For this review, take the finished solid that the model builds, in its own axes (mm). Face numbers are marked on the shaded views. A direction names the side the tool comes from. Give positions to 0.01 mm unless a question says otherwise; leave off trailing zeros. Order: outer loops, then holes, each group sorted by start corner. A loop starts at its lowest first (then second) coordinate and runs counter-clockwise, first axis right, second up.
Item 1: Consider section A-A (y = 10.75). Give the boundary of the cut face in (x, z).
Item 2: Consider section B-B (z = -9). Give the boundary of the cut face in (x, y).
Item 3: For probe 1 along X at (y, z) = (8.25, -6.5); probe 2 along Y at (x, z) = (3.1, -9); probe 3 along Z at (x, y) = (7, 10.3), list the stretches that pass through material, from the lowest coordinate up.
Item 4: Consider section C-C (x = 7). Give the boundary of the cut face in (y, z).
Item 5: For P1, Ø3, axis at x = 8.5, z = -3, coming from the -Y side; P2, Ø1.5, axis at y = 3, z = -18, coming from the +X side; P3, Ø1.2, axis at x = 6.5, y = 7.5, coming from the -Z side; P4, Ø1.2, axis at y = 3.5, z = -4, coming from the -X side, all flat-tipped, find the tip position at first contact; note any pin that passes through.
Item 6: The part is to be moulded in two halves that separate along Z. For the marked faces 1, 2 and 3, say which applies: released by +Z, released by -Z, zero draft, split by the parting line, or undercut.
Item 7: Consider section D-D (y = 3.5). Give the boundary of the cut face in (x, z).
Item 8: Machinability: for the marked faces 4, 5 and 6, which of the approach directions +Z, -Z, +X, -X, +Y, -Y give a long, thin tool a straight path to every point of the face, cutting with its end or side? Answer none if there is none.
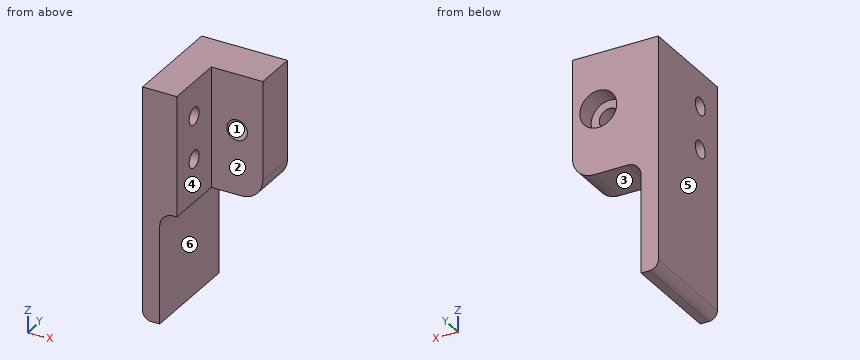
```python
from build123d import *

# Parameters (mm, degrees)
EXTRUDE_1_DEPTH              = 12
SKETCH_2_W                   = 6
SKETCH_2_H                   = 20
CUT_EXTRUDE_1_DEPTH          = 7
F_2_0MM_1_D                  = 2
HOLE_WIZARD_M2_1_D           = 2.4
HOLE_WIZARD_M2_1_CBORE_D     = 4.3
HOLE_WIZARD_M2_1_CBORE_DEPTH = 2.3


with BuildPart() as part:
    # 草图1 → 凸台-拉伸1 (new body)
    with BuildSketch(Plane(origin=(0, 0, 0), x_dir=(1, 0, 0), z_dir=(0, 1, 0))):
        with BuildLine():
            Line((3.6, 14), (7.5, 14))
            ThreePointArc((7.5, 14), (9.267766953, 13.267766953), (10, 11.5))
            Line((10, 11.5), (10, 0))
            Line((10, 0), (0, 0))
            Line((0, 0), (0, 26))
            ThreePointArc((0, 26), (0.292893219, 26.707106781), (1, 27))
            Line((1, 27), (2, 27))
            Line((2, 27), (2, 15.6))
            ThreePointArc((2, 15.6), (2.46862915, 14.46862915), (3.6, 14))
        make_face()
    extrude(amount=EXTRUDE_1_DEPTH)

    # 草图2 → 切除-拉伸1 (cut)
    with BuildSketch(Plane.XZ):
        with Locations((7, -10)):
            Rectangle(SKETCH_2_W, SKETCH_2_H)
    extrude(amount=-CUT_EXTRUDE_1_DEPTH, mode=Mode.SUBTRACT)

    # Ø2.0mm 暗销孔1 (through all)
    with Locations(Plane.ZY):
        with Locations((-4, 3.5), (-9, 3.5)):
            Hole(F_2_0MM_1_D / 2)

    # M2 六角圆柱头螺钉的柱形沉头孔1 (through all)
    with Locations(Plane(origin=(0, 12, 0), x_dir=(1, 0, 0), z_dir=(0, 1, 0))):
        with Locations((7, 6.5)):
            CounterBoreHole(HOLE_WIZARD_M2_1_D / 2, HOLE_WIZARD_M2_1_CBORE_D / 2, HOLE_WIZARD_M2_1_CBORE_DEPTH)


solid = part.part
```
Resolved:
1. outline: (0, -26) arc R1 ccw to (1, -27) - (2, -27) - (2, -15.6) arc R1.6 cw to (3.6, -14) - (7.5, -14) arc R2.5 ccw to (10, -11.5) - (10, 0) - (0, 0) - close; hole circle Ø4.3 at (7, -6.5)
2. outline: (0, 0) - (4, 0) - (4, 2.5) - (0, 2.5) - close; (0, 4.5) - (4, 4.5) - (4, 7) - (10, 7) - (10, 12) - (0, 12) - close
3. probe 1: x = 0 to 5.8, 8.2 to 10
3. probe 2: y = 0 to 2.5, 4.5 to 12
3. probe 3: z = -14 to -8.65, -4.35 to 0
4. outline: (7, -14) - (12, -14) - (12, -8.65) - (9.7, -8.65) - (9.7, -7.7) - (7, -7.7) - close; (7, -5.3) - (9.7, -5.3) - (9.7, -4.35) - (12, -4.35) - (12, 0) - (7, 0) - close
5. P1: stops at y = 7
5. P2: stops at x = 2
5. P3: stops at z = -14
5. P4: passes through
6. face 1: undercut
6. face 2: zero draft
6. face 3: released by -Z
7. outline: (0, -26) arc R1 ccw to (1, -27) - (2, -27) - (2, -15.6) arc R1.6 cw to (3.6, -14) - (4, -14) - (4, -10) - (0, -10) - close; (0, -8) - (4, -8) - (4, -5) - (0, -5) - close; (0, -3) - (4, -3) - (4, 0) - (0, 0) - close
8. face 4: +Z, -Z, +X, -Y
8. face 5: +Z, -Z, -X, +Y, -Y
8. face 6: -Z, +X, +Y, -Y
